```python
from build123d import *

# Parameters (mm, degrees)
SKETCH1_W           = 80
SKETCH1_H           = 80
BOSS_EXTRUDE1_DEPTH = 2.5
SKETCH3_W           = 80
SKETCH3_H           = 80
SKETCH3_W_2         = 75
SKETCH3_H_2         = 75
BOSS_EXTRUDE2_DEPTH = 12.5
BOSS_EXTRUDE3_DEPTH = 6.5
SKETCH5_W           = 13
SKETCH5_H           = 6
CUT_EXTRUDE1_DEPTH  = 58.933151131
CUT_EXTRUDE2_REACH  = 92.692
SKETCH6_W           = 32
SKETCH6_H           = 12.5
CUT_EXTRUDE3_REACH  = 92.692
SKETCH7_W           = 11.2
SKETCH7_H           = 7.2
BOSS_EXTRUDE4_DEPTH = 77.35
CUT_EXTRUDE4_REACH  = 92.692
BOSS_EXTRUDE5_REACH = 90.494
SKETCH15_W          = 2.5
SKETCH15_H          = 2
BOSS_EXTRUDE6_DEPTH = 2.5
SKETCH16_W          = 5
SKETCH16_H          = 12.5
SKETCH16_W_2        = 4
CUT_EXTRUDE5_DEPTH  = 1.25
SKETCH17_W          = 4
SKETCH17_H          = 1.5
BOSS_EXTRUDE7_DEPTH = 2
CUT_EXTRUDE7_REACH  = 92.692
SKETCH18_R          = 3.7
CUT_EXTRUDE8_REACH  = 92.692
SKETCH19_R          = 2.425


with BuildPart() as part:
    # Sketch1 → Boss-Extrude1 (new body)
    with BuildSketch(Plane(origin=(0, 0, 0), x_dir=(1, 0, 0), z_dir=(0, 1, 0))):
        Rectangle(SKETCH1_W, SKETCH1_H)
    extrude(amount=BOSS_EXTRUDE1_DEPTH)

    # Sketch3 → Boss-Extrude2 (add)
    with BuildSketch(Plane(origin=(0, 2.5, 0), x_dir=(1, 0, 0), z_dir=(0, 1, 0))):
        Rectangle(SKETCH3_W, SKETCH3_H)
        Rectangle(SKETCH3_W_2, SKETCH3_H_2, mode=Mode.SUBTRACT)
    extrude(amount=BOSS_EXTRUDE2_DEPTH)

    # Sketch2 → Boss-Extrude3 (add)
    with BuildSketch(Plane(origin=(0, 2.5, 0), x_dir=(1, 0, 0), z_dir=(0, 1, 0))):
        with BuildLine():
            ThreePointArc((-8.653956432, 23.98664291), (-6.354755269, 24.695487148), (-3.998981529, 25.184482261))
            Line((-3.998981529, 25.184482261), (-4.234215736, 26.665922394))
            ThreePointArc((-4.234215736, 26.665922394), (-6.862755968, 26.113264455), (-9.423377938, 25.302172797))
            Line((-9.423377938, 25.302172797), (-8.653956432, 23.98664291))
        make_face()
        with BuildLine():
            Line((4.234215736, 26.665922394), (3.998981529, 25.184482261))
            ThreePointArc((3.998981529, 25.184482261), (6.354755269, 24.695487148), (8.653956432, 23.98664291))
            Line((8.653956432, 23.98664291), (9.423377938, 25.302172797))
            ThreePointArc((9.423377938, 25.302172797), (6.862755968, 26.113264455), (4.234215736, 26.665922394))
        make_face()
        with BuildLine():
            Line((-8.653956432, -23.98664291), (-9.423377938, -25.302172797))
            ThreePointArc((-9.423377938, -25.302172797), (-6.862755968, -26.113264455), (-4.234215736, -26.665922394))
            Line((-4.234215736, -26.665922394), (-3.998981529, -25.184482261))
            ThreePointArc((-3.998981529, -25.184482261), (-6.354755269, -24.695487148), (-8.653956432, -23.98664291))
        make_face()
        with BuildLine():
            Line((9.423377938, -25.302172797), (8.653956432, -23.98664291))
            ThreePointArc((8.653956432, -23.98664291), (6.354755269, -24.695487148), (3.998981529, -25.184482261))
            Line((3.998981529, -25.184482261), (4.234215736, -26.665922394))
            ThreePointArc((4.234215736, -26.665922394), (6.862755968, -26.113264455), (9.423377938, -25.302172797))
        make_face()
    extrude(amount=BOSS_EXTRUDE3_DEPTH)

    # Sketch5 → Cut-Extrude1 (cut, through all)
    with BuildSketch(Plane(origin=(0, 2.5, 0), x_dir=(1, 0, 0), z_dir=(0, 1, 0))):
        with Locations((0, -30.5)):
            Rectangle(SKETCH5_W, SKETCH5_H)
    extrude(amount=-CUT_EXTRUDE1_DEPTH, mode=Mode.SUBTRACT)

    # Sketch6 → Cut-Extrude2 (cut, up to next)
    with BuildSketch(Plane.XY.offset(40), mode=Mode.PRIVATE) as cut_extrude2_sk1:
        with Locations((0, 8.75)):
            Rectangle(SKETCH6_W, SKETCH6_H)
    cut_extrude2_tool1 = extrude(cut_extrude2_sk1.sketch, amount=-CUT_EXTRUDE2_REACH, mode=Mode.PRIVATE) & part.part
    add(cut_extrude2_tool1.solids().sort_by_distance((0, 8.75, 40))[0], mode=Mode.SUBTRACT)

    # Sketch7 → Cut-Extrude3 (cut, up to next)
    with BuildSketch(Plane(origin=(0, 0, -40), x_dir=(-1, 0, 0), z_dir=(0, 0, -1)), mode=Mode.PRIVATE) as cut_extrude3_sk1:
        with Locations((0, 8.6)):
            Rectangle(SKETCH7_W, SKETCH7_H)
    cut_extrude3_tool1 = extrude(cut_extrude3_sk1.sketch, amount=-CUT_EXTRUDE3_REACH, mode=Mode.PRIVATE) & part.part
    add(cut_extrude3_tool1.solids().sort_by_distance((0, 8.6, -40))[0], mode=Mode.SUBTRACT)

    # Sketch9 → Boss-Extrude4 (add)
    with BuildSketch(Plane(origin=(0, 0, -40), x_dir=(-1, 0, 0), z_dir=(0, 0, -1))):
        Polygon((34.8, 0), (32.3, 0), (32.3, -4.3), (37.35, -4.3), (37.35, -2.3), (34.8, -2.3), align=None)
        Polygon((-32.3, 0), (-34.8, 0), (-34.8, -2.3), (-37.35, -2.3), (-37.35, -4.3), (-32.3, -4.3), align=None)
    extrude(amount=-BOSS_EXTRUDE4_DEPTH)

    # Sketch10 → Cut-Extrude4 (cut, up to next)
    with BuildSketch(Plane(origin=(0, 0, -40), x_dir=(-1, 0, 0), z_dir=(0, 0, -1)), mode=Mode.PRIVATE) as cut_extrude4_sk1:
        Polygon((-32.2, 15), (-35, 15), (-35, 13), (-37.5, 13), (-37.5, 10.7), (-32.2, 10.7), align=None)
    cut_extrude4_tool1 = extrude(cut_extrude4_sk1.sketch, amount=-CUT_EXTRUDE4_REACH, mode=Mode.PRIVATE) & part.part
    # Sketch10 → Cut-Extrude4 (cut, up to next)
    with BuildSketch(Plane(origin=(0, 0, -40), x_dir=(-1, 0, 0), z_dir=(0, 0, -1)), mode=Mode.PRIVATE) as cut_extrude4_sk2:
        Polygon((35, 15), (32.2, 15), (32.2, 10.7), (37.5, 10.7), (37.5, 13), (35, 13), align=None)
    cut_extrude4_tool2 = extrude(cut_extrude4_sk2.sketch, amount=-CUT_EXTRUDE4_REACH, mode=Mode.PRIVATE) & part.part
    add(cut_extrude4_tool1.solids().sort_by_distance((34.456521, 12.526785, -40))[0], mode=Mode.SUBTRACT)
    add(cut_extrude4_tool2.solids().sort_by_distance((-34.456521, 12.526785, -40))[0], mode=Mode.SUBTRACT)

    # Sketch15 → Boss-Extrude5 (add, up to next)
    with BuildSketch(Plane.XY.offset(-37.5), mode=Mode.PRIVATE) as boss_extrude5_sk1:
        with Locations((36.25, 14)):
            Rectangle(SKETCH15_W, SKETCH15_H)
    boss_extrude5_tool1 = extrude(boss_extrude5_sk1.sketch, amount=BOSS_EXTRUDE5_REACH, mode=Mode.PRIVATE) - part.part
    # Sketch15 → Boss-Extrude5 (add, up to next)
    with BuildSketch(Plane.XY.offset(-37.5), mode=Mode.PRIVATE) as boss_extrude5_sk2:
        with Locations((-36.25, 14)):
            Rectangle(SKETCH15_W, SKETCH15_H)
    boss_extrude5_tool2 = extrude(boss_extrude5_sk2.sketch, amount=BOSS_EXTRUDE5_REACH, mode=Mode.PRIVATE) - part.part
    add(boss_extrude5_tool1.solids().sort_by_distance((36.25, 14, -37.5))[0])
    add(boss_extrude5_tool2.solids().sort_by_distance((-36.25, 14, -37.5))[0])

    # Sketch2<3> → Boss-Extrude6 (add)
    with BuildSketch(Plane(origin=(0, 2.5, 0), x_dir=(1, 0, 0), z_dir=(0, 1, 0))):
        with BuildLine():
            ThreePointArc((18.5, 0), (0, 18.5), (-18.5, 0))
            Line((-18.5, 0), (0, 0))
            Line((0, 0), (0, -18.5))
            ThreePointArc((0, -18.5), (13.081475452, -13.081475452), (18.5, 0))
        make_face()
        with BuildLine():
            Line((0, 0), (-18.5, 0))
            ThreePointArc((-18.5, 0), (-13.081475452, -13.081475452), (0, -18.5))
            Line((0, -18.5), (0, 0))
        make_face()
    extrude(amount=BOSS_EXTRUDE6_DEPTH)

    # Sketch16 → Cut-Extrude5 (cut)
    with BuildSketch(Plane(origin=(0, 0, 37.5), x_dir=(-1, 0, 0), z_dir=(0, 0, -1))):
        with Locations((18.5, 8.75)):
            Rectangle(SKETCH16_W, SKETCH16_H)
        with Locations((-18, 8.75)):
            Rectangle(SKETCH16_W_2, SKETCH16_H)
    extrude(amount=-CUT_EXTRUDE5_DEPTH, mode=Mode.SUBTRACT)

    # Sketch17 → Boss-Extrude7 (add)
    with BuildSketch(Plane(origin=(0, 2.5, 0), x_dir=(1, 0, 0), z_dir=(0, 1, 0))):
        with Locations((-11.5, -35.25)):
            Rectangle(SKETCH17_W, SKETCH17_H)
        with Locations((11.5, -35.25)):
            Rectangle(SKETCH17_W, SKETCH17_H)
    extrude(amount=BOSS_EXTRUDE7_DEPTH)

    # Sketch18 → Cut-Extrude7 (cut, up to next)
    with BuildSketch(Plane(origin=(0, 0, -40), x_dir=(-1, 0, 0), z_dir=(0, 0, -1)), mode=Mode.PRIVATE) as cut_extrude7_sk1:
        with Locations((-22.5, 8.75)):
            Circle(SKETCH18_R)
    cut_extrude7_tool1 = extrude(cut_extrude7_sk1.sketch, amount=-CUT_EXTRUDE7_REACH, mode=Mode.PRIVATE) & part.part
    add(cut_extrude7_tool1.solids().sort_by_distance((22.5, 8.75, -40))[0], mode=Mode.SUBTRACT)

    # Sketch19 → Cut-Extrude8 (cut, up to next)
    with BuildSketch(Plane(origin=(0, 0, -40), x_dir=(-1, 0, 0), z_dir=(0, 0, -1)), mode=Mode.PRIVATE) as cut_extrude8_sk1:
        with Locations((25, 8.75)):
            Circle(SKETCH19_R)
    cut_extrude8_tool1 = extrude(cut_extrude8_sk1.sketch, amount=-CUT_EXTRUDE8_REACH, mode=Mode.PRIVATE) & part.part
    add(cut_extrude8_tool1.solids().sort_by_distance((-25, 8.75, -40))[0], mode=Mode.SUBTRACT)


solid = part.part
```
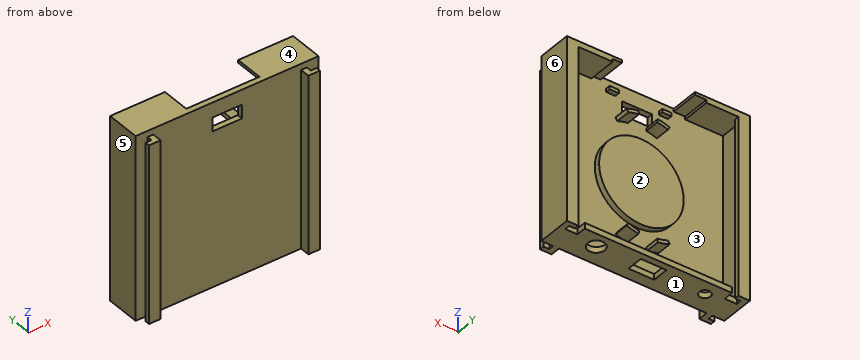
The model under review builds one solid part; all positions refer to its coordinate system, in mm. Face numbers are marked on the shaded views. A direction names the side the tool comes from. Round coordinates to 2 decimals unless told otherwise and drop trailing zeros. Order: outer loops, then holes, each group sorted by start corner. A loop starts at its lowest first (then second) coordinate and runs counter-clockwise, first axis right, second up. Notation, with made-up numbers: (-21, -19) -> (-5, -19) arc R22 ccw to (-5, 11) -> close; hole circle Ø8 at (48, 84.5). An arc over 180 degrees is marked (long way). Use a Markdown table: item, result.
Q1. For line 1 (Y direction, x = -25, z = -39.1) (3 decimals); line 2 (Y direction, x = 22.5, z = -38.3); line 3 (X direction, y = 13.25, z = 16), list the stretches that pass through material, from the lowest coordinate up.
Values:
| item | result |
|---|---|
| line 1 | y = 0 to 6.325, 11.175 to 15 |
| line 2 | y = 0 to 5.05, 12.45 to 15 |
| line 3 | x = -40 to -35, 35 to 40 |
Q2. We need section C-C on z = -33. Write out the cut boundary in (x, y).
Values:
| item | result |
|---|---|
| outline | (-40, 0) -> (-34.8, 0) -> (-34.8, -2.3) -> (-37.35, -2.3) -> (-37.35, -4.3) -> (-32.3, -4.3) -> (-32.3, 0) -> (32.3, 0) -> (32.3, -4.3) -> (37.35, -4.3) -> (37.35, -2.3) -> (34.8, -2.3) -> (34.8, 0) -> (40, 0) -> (40, 15) -> (35, 15) -> (35, 13) -> (37.5, 13) -> (37.5, 2.5) -> (-37.5, 2.5) -> (-37.5, 13) -> (-35, 13) -> (-35, 15) -> (-40, 15) -> close |
Q3. We need section B-B on x = 22.5. Write out the cut boundary in (y, z), then the cut area to 3 significant figures.
Values:
| item | result |
|---|---|
| outline | (0, -40) -> (5.05, -40) -> (5.05, -37.5) -> (2.5, -37.5) -> (2.5, 37.5) -> (15, 37.5) -> (15, 40) -> (0, 40) -> close; (12.45, -40) -> (15, -40) -> (15, -37.5) -> (12.45, -37.5) -> close |
| area | 244 mm^2 |
Q4. Mouldability with a two-part tool opening along X and no side actions: class the marked faces 3, 4, 5 and 6 as +X half, -X half, draft (parallel to the pull), parting line (faces both ways), or undercut.
Values:
| item | result |
|---|---|
| face 3 | undercut |
| face 4 | draft |
| face 5 | -X half |
| face 6 | +X half |
Q5. Tool access review of the marked faces 1 and 2: name each direction out of +Z, -Z, +X, -X, +Y, -Y from which nothing blocks a thin tool from reaching the whole face with its end or side.
Values:
| item | result |
|---|---|
| face 1 | -Z, +X, -X, +Y, -Y |
| face 2 | +Y |
Q6. Clearance check with flat-ended pins moving along their axes: P1, Ø2, axis at x = 3, z = 7, coming from the -Y side; P2, Ø1.2, axis at x = -11.5, z = 35.5, coming from the +Y side; P3, Ø6.5, axis at x = 22.5, y = 8.75, coming from the -Z side; P4, Ø1, axis at x = -2.5, y = 6.5, coming from the -Z side. State where each tip first meets the part, or that it passes through.
Values:
| item | result |
|---|---|
| P1 | stops at y = 0 |
| P2 | stops at y = 4.5 |
| P3 | stops at z = 37.5 |
| P4 | passes through |
Q7. We need section D-D on x = -25. Write out the cut boundary in (y, z) (3 decimals), then the cut area to 3 significant figures.
Values:
| item | result |
|---|---|
| outline | (0, -40) -> (6.325, -40) -> (6.325, -37.5) -> (2.5, -37.5) -> (2.5, 37.5) -> (15, 37.5) -> (15, 40) -> (0, 40) -> close; (11.175, -40) -> (15, -40) -> (15, -37.5) -> (11.175, -37.5) -> close |
| area | 250 mm^2 |
Q8. We need section A-A on y = -1.25. Write out the cut boundary in (x, z), then the cut area to 3 significant figures.
Values:
| item | result |
|---|---|
| outline | (-34.8, -40) -> (-32.3, -40) -> (-32.3, 37.35) -> (-34.8, 37.35) -> close; (32.3, -40) -> (34.8, -40) -> (34.8, 37.35) -> (32.3, 37.35) -> close |
| area | 387 mm^2 |
